Can you work these out from the model? Positions are in its coordinate system, mm. Face numbers are marked on the shaded views. Round coordinates to 2 decimals unless told otherwise and drop trailing zeros. Loops run counter-clockwise (first coordinate to the right, second up) from the corner with the lowest first, then second, coordinate; pieces in that order, holes last. Notation, with made-up numbers: (61.5, 22) -> (94.5, 22) arc R21 cw to (94.5, 30) -> close; hole circle Ø11 at (41.5, -8.5). An arc over 180 degrees is marked (long way). Answer as a JSON object with one key per item and string values.
```python
from build123d import *

# Parameters (mm, degrees)
BOSS_EXTRUDE1_DEPTH     = 120
CUT_EXTRUDE1_DEPTH      = 805.366061409
CUT_EXTRUDE1_DEPTH_BACK = 805.366061409
SKETCH2_R               = 10


with BuildPart() as part:
    # Sketch1 → Boss-Extrude1 (new body)
    with BuildSketch(Plane(origin=(0, 0, 0), x_dir=(1, 0, 0), z_dir=(0, 1, 0))):
        with BuildLine():
            Line((103.980664092, -784.528333178), (102.980664092, -774.578458807))
            ThreePointArc((102.980664092, -774.578458807), (23.980664092, -778.538383493), (-55.019335908, -774.578458807))
            Line((-55.019335908, -774.578458807), (-56.019335908, -784.528333178))
            ThreePointArc((-56.019335908, -784.528333178), (23.980664092, -788.538383493), (103.980664092, -784.528333178))
        make_face()
    extrude(amount=BOSS_EXTRUDE1_DEPTH)

    # Sketch2 → Cut-Extrude1 (cut, two sides: drawn at the far end of the back side and taken through both)
    with BuildSketch(Plane.XY.offset(-CUT_EXTRUDE1_DEPTH_BACK)):
        with Locations(Location((-31.019335908, 95, 0), (0, 0, 180))):
            Circle(SKETCH2_R)
        with Locations(Location((78.980664092, 95, 0), (0, 0, 180))):
            Circle(SKETCH2_R)
        with Locations(Location((78.980664092, 25, 0), (0, 0, 180))):
            Circle(SKETCH2_R)
        with Locations(Location((-31.019335908, 25, 0), (0, 0, 180))):
            Circle(SKETCH2_R)
    extrude(amount=CUT_EXTRUDE1_DEPTH + CUT_EXTRUDE1_DEPTH_BACK, mode=Mode.SUBTRACT)


solid = part.part
```
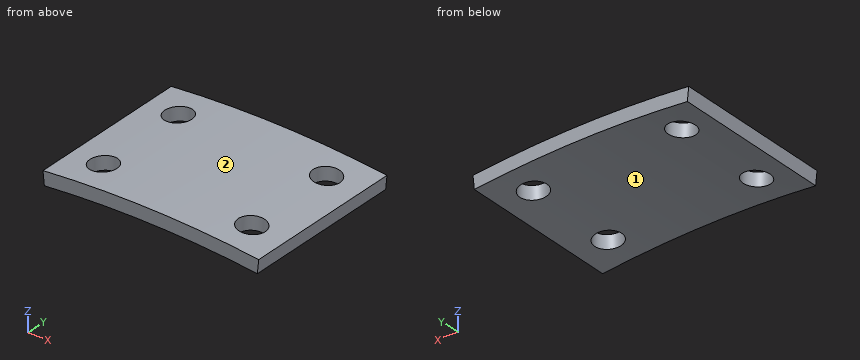
Q1. I want a section at C-C, the plane x = 23. Write out the boundary of the cut face in (y, z).
Determined:
{"outline": "(0, 778.54) -> (120, 778.54) -> (120, 788.54) -> (0, 788.54) -> close"}
Q2. I want a section at D-D, the plane x = -2.5. Write out the boundary of the cut face in (y, z).
Determined:
{"outline": "(0, 778.09) -> (120, 778.09) -> (120, 788.1) -> (0, 788.1) -> close"}
Q3. We'd pull the mould along X, two halves only. Please class the marked faces 1 and 2: pulls with the +X half, pulls with the -X half, needs draft (parallel to the pull), parting line crosses it, or undercut.
Determined:
{"face 1": "undercut", "face 2": "parting line crosses it"}
Q4. If I drill on L1, parallel to X at y = 25, z = 783.25; L2, parallel to Y at x = 84.5, z = 782.75; L3, parallel to X at y = 30, z = 779, over which ranges is the centre line in solid material (lowest first)? Write a range as [from, to].
Determined:
{"L1": "[-55.89, -41.02], [-21.02, 68.98], [88.98, 103.85]", "L2": "[0, 16.66], [33.34, 86.66], [103.34, 120]", "L3": "[-55.46, -39.68], [-22.36, 70.32], [87.64, 103.43]"}
Q5. I want a section at B-B, the plane y = 95. Write out the boundary of the cut face in (x, z), then the cut area to 3 significant figures.
Determined:
{"outline": "(-56.02, 784.53) -> (-55.02, 774.58) arc R790 cw to (-41.02, 775.86) -> (-41.02, 785.89) arc R800 ccw to start; (-21.02, 777.26) arc R790 cw to (68.98, 777.26) -> (68.98, 787.27) arc R800 ccw to (-21.02, 787.27) -> close; (88.98, 775.86) arc R790 cw to (102.98, 774.58) -> (103.98, 784.53) arc R800 ccw to (88.98, 785.89) -> close", "area": "1,190 mm²"}
Q6. I want a section at A-A, the plane x = 72.5. Write out the boundary of the cut face in (y, z), then the cut area to 3 significant figures.
Determined:
{"outline": "(0, 777.05) -> (17.38, 777.05) -> (17.38, 787.07) -> (0, 787.07) -> close; (32.62, 777.05) -> (87.38, 777.05) -> (87.38, 787.07) -> (32.62, 787.07) -> close; (102.62, 777.05) -> (120, 777.05) -> (120, 787.07) -> (102.62, 787.07) -> close", "area": "897 mm²"}
Q7. I'm going to push flat-ended pins straight in: pin 1 (18 mm diameter, centred on x = -31.02, y = 95, fed in from -Z); pin 2 (8 mm diameter, centred on y = 61.5, z = 779.5, fed in from -X); pin 3 (3 mm diameter, centred on y = 49, z = 778, fed in from -X); pin 4 (1.5 mm diameter, centred on y = 33.5, z = 778.5, fed in from +X). Where does each tip first touch, or does it pass through?
Determined:
{"pin 1": "through", "pin 2": "x = -55.92", "pin 3": "x = -55.51", "pin 4": "x = 103.45"}
